Input: part model. Units: mm. Frame: model coordinates. Face numbers are marked on the shaded views. A direction names the side the tool comes from. Coordinates: 2 decimals unless noted, no trailing zeros. Write each loop counter-clockwise with the first axis right and the second up, starting at its lowest first coordinate (ties: lowest second). Pieces come first, ordered by that corner, then holes. Notation, with made-up numbers: (-26.75, 50.5) - (-18.75, 50.5) arc R16 cw to (-18.75, 81.5) - close; hole circle Ø11 at (-10.75, 86). An arc over 180 degrees is marked (long way). One line per question, with ' | ' between items. Start each with the question number.
1) Section query C-C on y = -5.5. Return loops of the section in (x, z), and give its area (3 significant figures).
2) Section query A-A on x = 7.5. Return loops of the section in (y, z).
3) Line query: line 1 (Y direction, x = 6.5, z = 6.25); line 2 (X direction, y = 13.5, z = 6.5); line 3 (X direction, y = -9, z = 5.5). Output: solid intervals per line, ascending.
4) Reachability of the marked faces 4, 5 and 6 from +Z, -Z, +X, -X, +Y, -Y: full face, straight path, thin tool, end or side. Return the list, or none.
5) Draft query along Y for the marked faces 1, 2 and 3. Return one class per face: released by +Y, released by -Y, zero draft, split by the parting line, or undercut.
6) First-contact query: P1, Ø3, axis at x = -3.5, z = 5.5, coming from the -Y side; P2, Ø3, axis at y = 16, z = 3.5, coming from the -X side; P3, Ø4, axis at y = -4, z = 5.5, coming from the -X side; P4, Ø4, axis at x = -7.5, y = 3.5, coming from the +Z side. Flat tips, straight axial feed; report the tip coordinate or a pass-through.
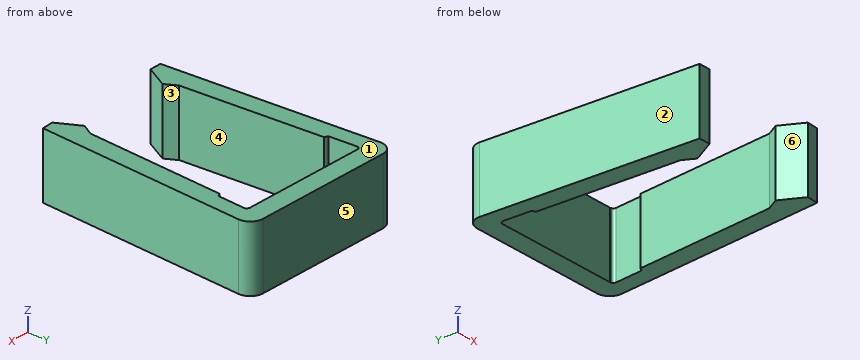
```python
from build123d import *

# Parameters (mm, degrees)
F1_DEPTH = 10


with BuildPart() as f1:
    # F0 (on Top) → F1 (new body)
    with BuildSketch(Plane.XY):
        with BuildLine():
            ThreePointArc((-10.218003, 18.066239), (-10.082748, 18.408666), (-9.75, 18.566239))
            Line((-9.75, 18.566239), (9.75, 18.566239))
            Line((9.75, 18.566239), (9.749928, 18.565147))
            ThreePointArc((9.749928, 18.565147), (10.093038, 18.395673), (10.215817, 18.03322))
            Line((10.215817, 18.03322), (9.937061, 13.821265))
            Line((9.937061, 13.821265), (9.419089, 13.566239))
            Line((9.419089, 13.566239), (8, -7.875915))
            Line((8, -7.875915), (7, -9.70099))
            Line((7, -9.70099), (8.880575, -13.133215))
            Line((8.880575, -13.133215), (10.666446, -13.015022))
            Line((10.666446, -13.015022), (12.814004, 19.434163))
            ThreePointArc((12.814004, 19.434163), (12.278533, 20.932959), (10.81837, 21.566239))
            Line((10.81837, 21.566239), (-10.81837, 21.566239))
            ThreePointArc((-10.81837, 21.566239), (-12.278533, 20.932959), (-12.814004, 19.434163))
            Line((-12.814004, 19.434163), (-10.658623, -13.133215))
            Line((-10.658623, -13.133215), (-8.866173, -13.133215))
            Line((-8.866173, -13.133215), (-7, -9.625915))
            Line((-7, -9.625915), (-8, -7.875915))
            Line((-8, -7.875915), (-9.419089, 13.566239))
            Line((-9.419089, 13.566239), (-9.937061, 13.821265))
            Line((-9.937061, 13.821265), (-10.218003, 18.066239))
        make_face()
    extrude(amount=F1_DEPTH)


solid = f1.part
```
Answer key:
1) outline: (-11.16, 0) - (-8.16, 0) - (-8.16, 10) - (-11.16, 10) - close; (8.16, 0) - (11.16, 0) - (11.16, 10) - (8.16, 10) - close | area: 60.1 mm²
2) outline: (-10.61, 0) - (-8.79, 0) - (-8.79, 10) - (-10.61, 10) - close; (18.57, 0) - (21.57, 0) - (21.57, 10) - (18.57, 10) - close
3) line 1: 18.57 to 21.57 | line 2: -12.42 to -9.41, 9.41 to 12.42 | line 3: -10.93 to -7.36, 7.38 to 10.93
4) face 4: +Z, -Z | face 5: +Z, -Z, +X, -X, +Y | face 6: +Z, -Z, -Y
5) face 1: zero draft | face 2: released by -Y | face 3: undercut
6) P1: y = 18.57 | P2: x = -12.69 | P3: x = -11.4 | P4: z = 10
